Input: part model. Units: mm. Frame: model coordinates. Face numbers are marked on the shaded views. A direction names the side the tool comes from. Give positions to 0.01 mm unless a question says otherwise; leave off trailing zeros. Order: outer loops, then holes, each group sorted by start corner. A loop starts at its lowest first (then second) coordinate and runs counter-clockwise, first axis right, second up. Notation, with made-up numbers: M 16.25,-11.5 L 69.25,-11.5 A18 ccw 69.25,-7.5 Z; hole C 47,20 d10. An arc over 180 degrees is marked long. Use a Markdown table: item, result.
Autodesk Inventor part; units mm, degrees
ref_plane "YZ Plane" through (0, 0, 0) normal (1, 0, 0) x (0, 1, 0)
ref_plane "XZ Plane" through (0, 0, 0) normal (0, 1, 0) x (-1, 0, 0)
ref_plane "XY Plane" through (0, 0, 0) normal (0, 0, 1) x (1, 0, 0)
sketch "Sketch1" plane through (0, 0, 0) normal (0, 0, 1) x (1, 0, 0)
  circle A0 centre (0, 0) radius 19.05
  dimension "d0" = 38.1
extrude "Extrusion1" add sketch "Sketch1" along normal blind 12.7
sketch "Sketch2" plane through (0, 0, 0) normal (0, 0, -1) x (-1, 0, 0)
  circle A0 centre (0, 0) radius 19.05
  line L0 (-17.9605, 6.35) -> (17.9605, 6.35)
  line L1 (17.9605, 6.35) -> (17.9605, -6.35)
  line L2 (17.9605, -6.35) -> (-17.9605, -6.35)
  line L3 (-17.9605, -6.35) -> (-17.9605, 6.35)
  dimension "d3" = 12.7
  dimension "d4" = 12.7
extrude "Extrusion2" add sketch "Sketch2" along normal blind 50.8 contours L1 L2 L3 L0
sketch "Sketch3" plane through (-17.9605, 6.35, 0) normal (0, 1, 0) x (1, 0, 0)
  circle A0 centre (17.9605, 38.1) radius 3.175
  line L0 (35.921, 0) -> (35.921, 50.8)
  line L1 (0, 50.8) -> (35.921, 50.8)
  point P0 (17.9605, 0)
  dimension "d7" = 6.35
  dimension "d8" = 17.9605
  dimension "d9" = 12.7
extrude "Extrusion3" cut sketch "Sketch3" against normal blind 25.4
properties part number "Bottom Pneumatics notch"
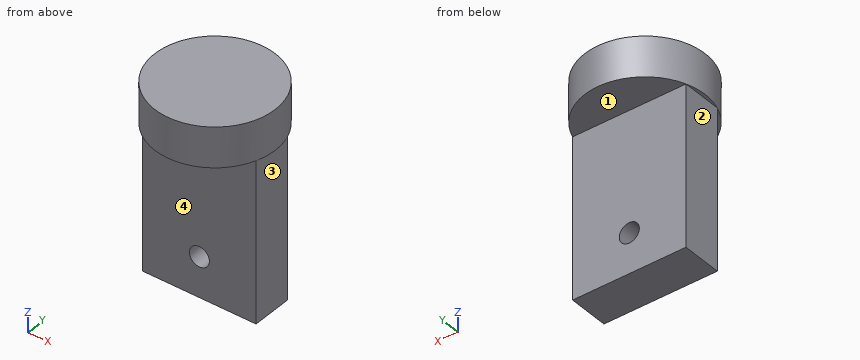
1) Cut plane D-D on z = 4.5. Return loops of the section in (x, y), and give its area (3 significant figures).
Response values:
| item | result |
|---|---|
| outline | C 0,0 d38.1 |
| area | 1,140 mm² |
2) First-contact query: pin 1 Ø0.5 at (x, y) = (18.5, 2.5) entering from -Z; pin 2 Ø5 at (y, z) = (0.5, -7) entering from +X; pin 3 Ø4 at (y, z) = (-3.5, 1.5) entering from +X. Flat tips, straight axial feed; report the tip coordinate or a pass-through.
Response values:
| item | result |
|---|---|
| pin 1 | stops at z = 0 |
| pin 2 | stops at x = 17.96 |
| pin 3 | stops at x = 18.99 |
3) Reachability of the marked faces 1, 2, 3 and 4 from +Z, -Z, +X, -X, +Y, -Y: full face, straight path, thin tool, end or side. Return the list, or none.
Response values:
| item | result |
|---|---|
| face 1 | -Z, +X, -X, +Y |
| face 2 | -Z, -X, +Y, -Y |
| face 3 | -Z, +X, +Y, -Y |
| face 4 | -Z, +X, -X, -Y |
4) Material intervals for line 1 (X direction, y = 1.5, z = -38.1) (1 decimal); line 2 (Z direction, x = 0, y = -1) (3 decimals); line 3 (Y direction, x = 15.5, z = -2.5), sorted ascending. Write a range as from..to.
Response values:
| item | result |
|---|---|
| line 1 | x = -18..-3.2, 3.2..18 |
| line 2 | z = -50.8..-41.275, -34.925..12.7 |
| line 3 | y = -6.35..6.35 |
5) Cut plane A-A on x = 0. Return loops of the section in (y, z) (3 decimals), and give its area (3 significant figures).
Response values:
| item | result |
|---|---|
| outline | M -19.05,0 L -6.35,0 L -6.35,-34.925 L 6.35,-34.925 L 6.35,0 L 19.05,0 L 19.05,12.7 L -19.05,12.7 Z; M -6.35,-50.8 L 6.35,-50.8 L 6.35,-41.275 L -6.35,-41.275 Z |
| area | 1,050 mm² |
